```python
from build123d import *

# Parameters (mm, degrees)
SKETCH_1_W      = 6
SKETCH_1_H      = 6
EXTRUDE_1_DEPTH = 3.1
SKETCH_2_R      = 1.75
EXTRUDE_2_DEPTH = 3.6
SKETCH_8_W      = 1.302494735
SKETCH_8_H      = 0.403244053
SKETCH_8_W_2    = 1.3
SKETCH_3_R      = 0.65
SKETCH_3_R_2    = 0.651247367
EXTRUDE_5_DEPTH = 0.55
FILLET_1_R      = 0.2
FILLET_2_R      = 0.2
FILLET_3_R      = 0.2
FILLET_4_R      = 0.2
SKETCH_13_W     = 1.29992486
SKETCH_13_H     = 0.404320481
SKETCH_13_W_2   = 1.3


with BuildPart() as part:
    # Эскиз1 → Бобышка-Вытянуть1 (new body)
    with BuildSketch(Plane(origin=(0, 0, 0), x_dir=(1, 0, 0), z_dir=(0, 1, 0))):
        Rectangle(SKETCH_1_W, SKETCH_1_H)
    extrude(amount=EXTRUDE_1_DEPTH)

    # Эскиз2 → Бобышка-Вытянуть2 (add)
    with BuildSketch(Plane(origin=(0, 3.1, 0), x_dir=(1, 0, 0), z_dir=(0, 1, 0))):
        with Locations(Location((0, 0, 0), (0, 0, 90))):
            Circle(SKETCH_2_R)
    extrude(amount=EXTRUDE_2_DEPTH)

    # По траектории11: sweep along a path in Эскиз11
    with BuildLine(Plane.XY) as sweep_11_path:
        Line((-3, 0.80118086), (-3.3, 0.80118086))
        ThreePointArc((-3.3, 0.80118086), (-3.512132034, 0.713312895), (-3.6, 0.50118086))
        Line((-3.6, 0.50118086), (-3.6, -1.49881914))
    # Эскиз8 → По траектории11 (sweep)
    with BuildSketch(Plane.ZY.offset(3)):
        with Locations((-2.002333521, 0.801180861)):
            Rectangle(SKETCH_8_W, SKETCH_8_H)
        with Locations((2.004025026, 0.801180861)):
            Rectangle(SKETCH_8_W_2, SKETCH_8_H)
    sweep(path=sweep_11_path.line)

    # Эскиз3 → Бобышка-Вытянуть5 (add)
    with BuildSketch(Plane(origin=(0, 3.1, 0), x_dir=(1, 0, 0), z_dir=(0, 1, 0))):
        with Locations(Location((-2.004298807, -2.004025026, 0), (0, 0, 90))):
            Circle(SKETCH_3_R)
        with Locations(Location((-2.004298807, 2.002333521, 0), (0, 0, 90))):
            Circle(SKETCH_3_R_2)
        with Locations(Location((2.001283613, 2.002333521, 0), (0, 0, 90))):
            Circle(SKETCH_3_R)
        with Locations(Location((2.001283613, -2.004025026, 0), (0, 0, 90))):
            Circle(SKETCH_3_R)
    extrude(amount=EXTRUDE_5_DEPTH)

    # Скругление1
    fillet_1_edges = [part.edges().sort_by_distance(p)[0] for p in [
        (2.001283613, 3.65, 2.654025026),
    ]]
    fillet(fillet_1_edges, radius=FILLET_1_R)

    # Скругление2
    fillet_2_edges = [part.edges().sort_by_distance(p)[0] for p in [
        (-2.004298807, 3.65, 2.654025026),
    ]]
    fillet(fillet_2_edges, radius=FILLET_2_R)

    # Скругление3
    fillet_3_edges = [part.edges().sort_by_distance(p)[0] for p in [
        (2.001283613, 3.65, -1.352333521),
    ]]
    fillet(fillet_3_edges, radius=FILLET_3_R)

    # Скругление4
    fillet_4_edges = [part.edges().sort_by_distance(p)[0] for p in [
        (-2.004298807, 3.65, -1.351086153),
    ]]
    fillet(fillet_4_edges, radius=FILLET_4_R)

    # По траектории12: sweep along a path in Эскиз14
    with BuildLine(Plane.XY) as sweep_12_path:
        Line((3, 0.793292299), (3.29676564, 0.793292299))
        ThreePointArc((3.29676564, 0.793292299), (3.508897675, 0.705424334), (3.59676564, 0.493292299))
        Line((3.59676564, 0.493292299), (3.59676564, -1.507497103))
    # Эскиз13 → По траектории12 (sweep)
    with BuildSketch(Plane(origin=(3, 0, 0), x_dir=(0, 0, -1), z_dir=(1, 0, 0))):
        with Locations((-2.004083718, 0.7932923)):
            Rectangle(SKETCH_13_W, SKETCH_13_H)
        with Locations((2.002333521, 0.7932923)):
            Rectangle(SKETCH_13_W_2, SKETCH_13_H)
    sweep(path=sweep_12_path.line)


solid = part.part
```
Geometry: final body of the model. Coordinates: model frame, mm. A direction names the side the tool comes from. Round coordinates to 2 decimals unless told otherwise and drop trailing zeros. Write each loop counter-clockwise with the first axis right and the second up, starting at its lowest first coordinate (ties: lowest second). Pieces come first, ordered by that corner, then holes. Notation, with made-up numbers: (48.25, 27) -> (106.25, 27) arc R24 cw to (106.25, 61) -> close; hole circle Ø1 at (7, 62.5). An arc over 180 degrees is marked (long way). Use CSV: the item, a comma, the result in double quotes. Start each with the question number.
Q1. Pull-direction query (Z, two-part tool) for faces 1 (the face through (0, 2, -3)), 2 (the face through (0, 2, 3)), 3 (the face through (-1.4, 3.1, -1.4)), 4 (the face through (-2, 3.65, 2)); classes: pulls with the +Z half, pulls with the -Z half, needs draft (parallel to the pull), parting line crosses it, or undercut.
Q2. Section D-D (y = 5.5). Return loops of the section in (x, z).
Q3. Section A-A (x = 0). Return loops of the section in (y, z), plus the area to 3 significant figures.
Q4. Line query: L1, parallel to Z at x = -1.5, y = 3.5; L2, parallel to Y at x = 0, z = -1.95; L3, parallel to Z at x = -2.25, y = 3.5. Output: solid intervals per line, ascending.
Q5. Reachability of faces 5 (the face through (-3.398, -1, 2)), 6 (the face through (-2, 3.65, -2)), 7 (the face through (-3.6, -0.2, 1.354)) from +Z, -Z, +X, -X, +Y, -Y: full face, straight path, thin tool, end or side. Return the list, or none.
Q6. First-contact query: pin 1 Ø0.9 at (x, y) = (3.5, 0) entering from +Z; pin 2 Ø0.5 at (x, z) = (-2, -2) entering from +Y; pin 3 Ø2 at (y, z) = (2.5, -1.5) entering from +X. Flat tips, straight axial feed; report the tip coordinate or a pass-through.
Q7. Section B-B (z = 0). Return loops of the section in (x, y).
Q8. Section C-C (y = 2.5). Return loops of the section in (x, z), plus the area to 3 significant figures.
Result sheet:
1,face 1,"pulls with the -Z half"
1,face 2,"pulls with the +Z half"
1,face 3,"undercut"
1,face 4,"needs draft"
2,outline,"circle Ø3.5 at (0, 0)"
3,outline,"(0, -3) -> (3.1, -3) -> (3.1, -1.75) -> (6.7, -1.75) -> (6.7, 1.75) -> (3.1, 1.75) -> (3.1, 3) -> (0, 3) -> close"
3,area,"31.2 mm²"
4,L1,"-2.4 to -1.6, -0.9 to 0.9, 1.6 to 2.4"
4,L2,"0 to 3.1"
4,L3,"-2.6 to -1.41, 1.41 to 2.6"
5,face 5,"+Z, -Z, -Y"
5,face 6,"-Z, -X, +Y"
5,face 7,"-X, +Y, -Y"
6,pin 1,"z = 2.65"
6,pin 2,"y = 3.65"
6,pin 3,"x = 3"
7,outline,"(-3, 0) -> (3, 0) -> (3, 3.1) -> (1.75, 3.1) -> (1.75, 6.7) -> (-1.75, 6.7) -> (-1.75, 3.1) -> (-3, 3.1) -> close"
8,outline,"(-3, -3) -> (3, -3) -> (3, 3) -> (-3, 3) -> close"
8,area,"36.0 mm²"
